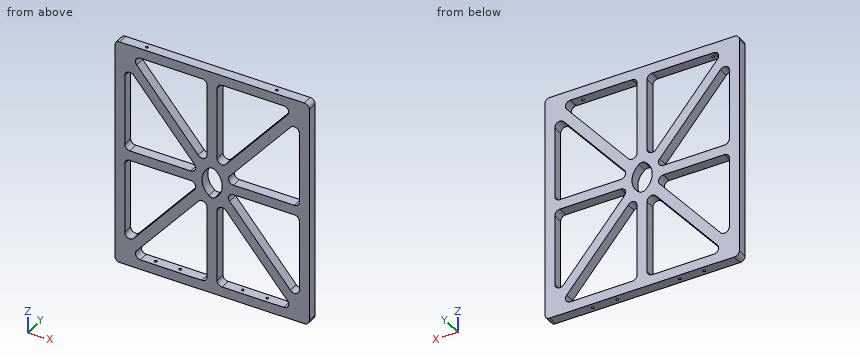
Autodesk Inventor part; units mm, degrees
ref_plane "YZ Plane" through (0, 0, 0) normal (1, 0, 0) x (0, 1, 0)
ref_plane "XZ Plane" through (0, 0, 0) normal (0, 1, 0) x (-1, 0, 0)
ref_plane "XY Plane" through (0, 0, 0) normal (0, 0, 1) x (1, 0, 0)
sketch "Sketch1" plane through (0, 0, 0) normal (0, 1, 0) x (-1, 0, 0)
  line L0 (0, 0) -> (389, 0)
  line L1 (389, 0) -> (389, -464)
  line L2 (389, -464) -> (0, -464)
  line L3 (0, -464) -> (0, 0)
  line L4 (369, -444) -> (369, -20)
  line L5 (369, -20) -> (20, -20)
  line L6 (20, -20) -> (20, -444)
  line L7 (20, -444) -> (369, -444)
  line L8 (184.5, 0) -> (204.5, 0)
  line L9 (204.5, 0) -> (204.5, -464)
  line L10 (204.5, -464) -> (184.5, -464)
  line L11 (184.5, -464) -> (184.5, 0)
  line L12 (0, -222) -> (389, -222)
  line L13 (389, -222) -> (389, -242)
  line L14 (389, -242) -> (0, -242)
  line L15 (0, -242) -> (0, -222)
  line L16 (396.6632, -6.4246) -> (7.6632, -470.4246)
  line L17 (381.3368, 6.4246) -> (-7.6632, -457.5754)
  line L18 (7.6632, 6.4246) -> (396.6632, -457.5754)
  line L19 (-7.6632, -6.4246) -> (381.3368, -470.4246)
  point P0 (369, -222)
  point P1 (215.933, -222)
  point P2 (369, -39.4213)
  point P3 (369, -242)
  point P4 (369, -424.5787)
  point P5 (215.933, -242)
  point P6 (184.5, -20)
  point P7 (184.5, -204.5067)
  point P8 (29.8166, -20)
  point P9 (20, -424.5787)
  point P10 (20, -242)
  point P11 (173.067, -242)
  point P12 (204.5, -259.4933)
  point P13 (359.1834, -444)
  point P14 (204.5, -444)
  point P15 (20, -39.4213)
  point P16 (173.067, -222)
  point P17 (20, -222)
  point P18 (359.1834, -20)
  point P19 (204.5, -204.5067)
  point P20 (204.5, -20)
  point P21 (184.5, -444)
  point P22 (29.8166, -444)
  point P23 (184.5, -259.4933)
  dimension "d0" = 389
  dimension "d1" = 464
  dimension "d2" = 20
  dimension "d3" = 20
  dimension "d4" = 20
extrude "Extrusion1" add sketch "Sketch1" along normal blind 20 contours L11 L5 L18 L0 | L0 L9 L5 L11 | L0 L17 L5 L9 | L18 L5 L6 L19 L3 L0 | L5 L9 L17 L18 L11 | L0 L1 L16 L4 L5 L17 | L18 L11 L12 L19 L6 L5 | L18 L17 L12 L11 | L5 L4 L16 L12 L9 L17 | L9 L12 L18 L17 | L19 L6 L12 L3 | L12 L17 L11 | L11 L17 L19 L12 | L18 L12 L17 | L1 L12 L4 L16 | L12 L16 L18 L9 | L9 L18 L12 | L12 L6 L14 L3 | L17 L12 L18 L9 L16 L14 L19 L11 | L11 L19 L17 | L19 L17 L14 L6 L12 | L1 L14 L4 L12 | L18 L16 L9 | L12 L4 L14 L18 L16 | L14 L6 L17 L3 | L19 L14 L11 | L11 L14 L17 L19 | L1 L18 L4 L14 | L16 L18 L14 L9 | L9 L14 L16 | L17 L6 L7 L16 L2 L3 | L14 L19 L16 L11 | L11 L16 L7 L6 L17 L14 | L14 L16 L19 | L1 L2 L19 L7 L4 L18 | L14 L18 L4 L7 L19 L9 | L9 L19 L16 L14 | L16 L19 L9 L7 L11 | L16 L7 L11 L2 | L7 L9 L2 L11 | L2 L9 L7 L19
fillet "Fillet1" radius 10 28 edges at (-389, 10, 0) (0, 10, 0) (0, 10, -464) (-389, 10, -464) (-369, 10, -424.5787) (-359.1834, 10, -444) (-369, 10, -242) (-369, 10, -222) (-204.5, 10, -444) (-204.5, 10, -259.4933) (-215.933, 10, -242) (-215.933, 10, -222) (-204.5, 10, -204.5067) (-184.5, 10, -204.5067) (-173.067, 10, -222) (-173.067, 10, -242) (-184.5, 10, -259.4933) (-369, 10, -39.4213) (-359.1834, 10, -20) (-204.5, 10, -20) (-184.5, 10, -20) (-29.8166, 10, -20) (-20, 10, -39.4213) (-20, 10, -222) (-20, 10, -242) (-20, 10, -424.5787) (-29.8166, 10, -444) (-184.5, 10, -444)
sketch "Sketch2" plane through (0, 20, 0) normal (0, 1, 0) x (1, 0, 0)
  line L0 (-389, 454) -> (-389, 10)
  line L1 (-389, 232) -> (0, 232)
  line L2 (0, 10) -> (0, 454)
  line L3 (-379, 0) -> (-10, 0)
  line L4 (-194.5, 0) -> (-194.5, 464)
  line L5 (-10, 464) -> (-379, 464)
  arc A0 (-194.5, 265) -> (-194.5, 199) centre (-177.7668, 232) ccw
  arc A1 (-194.5, 199) -> (-194.5, 265) centre (-211.2332, 232) ccw
  point P0 (0, 0)
  dimension "d12" = 66
  dimension "d13" = 37
  dimension "d14" = 37
extrude "Extrusion2" cut sketch "Sketch2" against normal through all
fillet "Fillet2" radius 10 2 edges at (-194.5, 10, -265) (-194.5, 10, -199)
sketch "Sketch6" plane through (-10, 0, -464) normal (0, 0, -1) x (-1, 0, 0)
  line L0 (369, 20) -> (369, 0)
  line L1 (0, 20) -> (369, 20)
  line L2 (0, 0) -> (0, 20)
  line L3 (0, 0) -> (369, 0)
  line L4 (0, 10) -> (80, 10)
  line L5 (0, 10) -> (80, 10) construction
  line L6 (80, 10) -> (129, 10)
  line L7 (369, 10) -> (303.0267, 10)
  line L8 (369, 10) -> (434.9733, 10) construction
  line L9 (303.0267, 10) -> (254.0267, 10)
  dimension "d48" = 80
  dimension "d49" = 0
  dimension "d50" = 49
  dimension "d51" = 180
  dimension "d52" = 180
  dimension "d53" = 49
  dimension "d54" = 180
hole "Hole2" at (-90, 10, -464) at (-139, 10, -464) at (-264.0267, 10, -464) at (-313.0267, 10, -464) direction (0, 0, 1) diameter 4.917 depth 20
sketch "Sketch8" plane through (-379, 0, 0) normal (0, 0, 1) x (1, 0, 0)
  line L0 (379, 0) -> (379, 20)
  line L1 (369, 20) -> (369, 0)
  line L2 (0, 20) -> (369, 20)
  line L3 (0, 0) -> (0, 20)
  line L4 (0, 0) -> (369, 0)
  line L5 (0, 10) -> (369, 10)
  line L6 (178.3025, 0) -> (178.3025, 20)
  line L7 (178.3025, 10) -> (308.3025, 10)
  line L8 (308.3025, 10) -> (48.3025, 10)
  dimension "d46" = 130
  dimension "d47" = 260
hole "Hole3" at (-330.6975, 10, 0) at (-70.6975, 10, 0) direction (0, 0, -1) diameter 4.917 depth 20
properties part number "Halterung_Aufbau"
Could you check a few things on this model? Use its own coordinates, in mm. Round coordinates to 2 decimals unless told otherwise and drop trailing zeros. Order: outer loops, then holes, each group sorted by start corner. A loop starts at its lowest first (then second) coordinate and runs counter-clockwise, first axis right, second up.
(1) Imagine slicing it at A-A (x = -102). Write out the boundary of the cut face in (y, z).
Response values:
outline: (0, -464) - (20, -464) - (20, -444) - (0, -444) - close; (0, -357.9) - (20, -357.9) - (20, -326.77) - (0, -326.77) - close; (0, -242) - (20, -242) - (20, -222) - (0, -222) - close; (0, -137.23) - (20, -137.23) - (20, -106.1) - (0, -106.1) - close; (0, -20) - (20, -20) - (20, 0) - (0, 0) - close
(2) Please list where these lines run through material, in increasing order: line 1 along X through (y, z) = (10, -448.75); line 2 along X through (y, z) = (8, -433); line 3 along X through (y, z) = (12, -374).
Response values:
line 1: x = -389 to -315.49, -310.57 to -266.49, -261.57 to -141.46, -136.54 to -92.46, -87.54 to 0
line 2: x = -389 to -347.7, -204.5 to -184.5, -41.3 to 0
line 3: x = -389 to -369, -326.6 to -300.5, -204.5 to -184.5, -88.5 to -62.4, -20 to 0
(3) I'm going to push a flat-ended pin straight in: pin 1 (3 mm diameter, centred on x = -313.03, y = 10, fed in from -Z). Where does the tip first touch, or does it pass through?
Response values:
pin 1: stops at z = -390.74
(4) Imagine slicing it at B-B (z = -328.5). Write out the boundary of the cut face in (x, y), plus the area to 3 significant figures.
Response values:
outline: (-389, 0) - (-369, 0) - (-369, 20) - (-389, 20) - close; (-288.45, 0) - (-262.35, 0) - (-262.35, 20) - (-288.45, 20) - close; (-204.5, 0) - (-184.5, 0) - (-184.5, 20) - (-204.5, 20) - close; (-126.65, 0) - (-100.55, 0) - (-100.55, 20) - (-126.65, 20) - close; (-20, 0) - (0, 0) - (0, 20) - (-20, 20) - close
area: 2,240 mm2
